Geometry: final body of the model. Coordinates: model frame, mm. A direction names the side the tool comes from. Round coordinates to 2 decimals unless told otherwise and drop trailing zeros. Order: outer loops, then holes, each group sorted by start corner. A loop starts at its lowest first (then second) coordinate and runs counter-clockwise, first axis right, second up. Notation, with made-up numbers: (-3, 28.5) - (24, 28.5) arc R19 ccw to (24, 63.5) - close; hole circle Ø8 at (-33.75, -24). An arc over 180 degrees is marked (long way). Put each result on its own line as item: value. Start each with the question number.
(1) Section B-B (z = 38). Output: boundary loops of the cut face in (x, y), and give its area (3 significant figures).
(2) Section C-C (z = 94). Output: boundary loops of the cut face in (x, y).
(3) Material intervals for L1, parallel to Z at x = 0.85, y = 9.5; L2, parallel to Y at x = 0.55, z = 2.5; L3, parallel to Y at x = 1.45, z = 10, sorted ascending. Write a range as [from, to].
(4) Section D-D (x = 0.8). Count the separate pieces of the cut face and the enclosed holes in it, and give its area (3 significant figures).
(5) Pin query (flat end, axial travel): P1, Ø1.3, axis at x = 1, z = 83, coming from the +Y side; P2, Ø0.8, axis at x = 1, z = 29, coming from the +Y side; P3, Ø0.8, axis at x = 1.5, z = 72, coming from the -Y side. Return the tip coordinate at first contact, or that it passes through.
(6) Access query for faces 1 (the face through (1, 32.105, 83)), 2 (the face through (1, -24, -3.819)), 3 (the face through (1, 33.231, 82)), 4 (the face through (1, -28, 21.581)). Directions: +Z, -Z, +X, -X, +Y, -Y. A direction counts if a zero-diameter tool reaches every point of the face in a straight line with its end or side. Return the directions, or none.
(7) Pull-direction query (Y, two-part tool) for faces 5 (the face through (1.288, 30.863, 106.352)), 6 (the face through (0, -39, 86)), 7 (the face through (1.252, 33.159, -2.864)); classes: released by +Y, released by -Y, zero draft, split by the parting line, or undercut.
(8) Section A-A (y = -12.5). Output: boundary loops of the cut face in (x, z), and give its area (3 significant figures).
Autodesk Inventor part; units mm, degrees
ref_plane "YZ Plane" through (0, 0, 0) normal (1, 0, 0) x (0, 1, 0)
ref_plane "XZ Plane" through (0, 0, 0) normal (0, 1, 0) x (-1, 0, 0)
ref_plane "XY Plane" through (0, 0, 0) normal (0, 0, 1) x (1, 0, 0)
sketch "Sketch1" plane through (0, 0, 0) normal (1, 0, 0) x (0, 1, 0)
  circle A0 centre (30.8347, 52.4486) radius 6.35
  line L0 (34.0644, 46.9813) -> (34.0644, -0.6437)
  line L1 (33.2311, 58.3291) -> (33.2311, 105.9541)
  line L2 (30.0561, 109.1291) -> (27.0711, 109.1291)
  arc A1 (33.2311, 105.9541) -> (30.0561, 109.1291) centre (30.0561, 105.9541) ccw
  line L3 (30.8894, -3.8187) -> (26.3644, -3.8187)
  arc A2 (30.8894, -3.8187) -> (34.0644, -0.6437) centre (30.8894, -0.6437) ccw
  line L4 (27.0711, 109.1291) -> (27.0711, 57.5631)
  line L5 (26.3644, -3.8187) -> (26.3644, 47.9388)
  line L6 (27.0711, 109.1291) -> (27.0711, 83.7291)
  line L7 (27.0711, 109.1291) -> (-79.6089, 109.1291)
  line L8 (-79.6089, 109.1291) -> (-79.6089, 83.7291)
  line L9 (-79.6089, 83.7291) -> (27.0711, 83.7291)
  line L10 (26.3644, -3.8187) -> (-80.3156, -3.8187)
  line L11 (-80.3156, -3.8187) -> (-80.3156, 21.5813)
  line L12 (26.3644, -3.8187) -> (26.3644, 21.5813)
  line L13 (26.3644, 21.5813) -> (-80.3156, 21.5813)
  circle A3 centre (30.8347, 52.4486) radius 4.7025
  point P0 (34.0644, -3.8187)
  point P1 (33.2311, 109.1291)
  dimension "d3" = 50.8
  dimension "d4" = 50.8
  dimension "d5" = 6.16
  dimension "d6" = 3.175
  dimension "d7" = 3.175
  dimension "d8" = 25.4
  dimension "d9" = 106.68
  dimension "d10" = 106.68
  dimension "d11" = 25.4
  dimension "d13" = 25.4
  dimension "d46" = 12.7
extrude "Extrusion1" add sketch "Sketch1" along normal blind 2.54 contours A0 | A0 L4 L2 A1 L1 | L0 A2 L3 L5 A0
sketch "Sketch2" plane through (2.54, 0, 0) normal (1, 0, 0) x (0, 0, -1)
  line L0 (-109.1291, 27.0711) -> (-57.5631, 27.0711)
  line L1 (-109.1291, 27.0711) -> (-109.1291, -79.6089)
  line L2 (-109.1291, -79.6089) -> (-83.7291, -79.6089)
  line L3 (-83.7291, -79.6089) -> (-83.7291, 27.0711)
  line L4 (-109.1291, 27.0711) -> (-83.7291, 27.0711)
  line L5 (3.8187, 26.3644) -> (3.8187, 30.8894)
  line L6 (3.8187, 26.3644) -> (3.8187, -80.3156)
  line L7 (3.8187, -80.3156) -> (-21.5813, -80.3156)
  line L8 (-21.5813, -80.3156) -> (-21.5813, 26.3644)
  line L9 (-47.9388, 26.3644) -> (3.8187, 26.3644)
  point P0 (0, 0)
  dimension "d16" = 106.68
  dimension "d17" = 25.4
  dimension "d18" = 106.68
  dimension "d19" = 25.4
extrude "Extrusion2" add sketch "Sketch2" against normal up to surface (2.54 mm away)
sketch "Sketch3" plane through (2.54, 0, 0) normal (1, 0, 0) x (0, 0, -1)
  line L0 (-83.7291, -79.6089) -> (-83.7291, 27.0711)
  line L1 (-58.3291, 33.2311) -> (-105.9541, 33.2311)
  line L2 (-109.1291, 30.0561) -> (-109.1291, -79.6089)
  line L3 (-109.1291, -79.6089) -> (-83.7291, -79.6089)
  line L4 (-96.4291, 20.7211) -> (-96.4291, 20.7211)
  line L5 (-90.0791, 14.3711) -> (-90.0791, -66.9089)
  line L6 (-96.4291, -73.2589) -> (-96.4291, -73.2589)
  line L7 (-102.7791, -66.9089) -> (-102.7791, 14.3711)
  arc A0 (-96.4291, 20.7211) -> (-102.7791, 14.3711) centre (-96.4291, 14.3711) ccw
  arc A1 (-90.0791, 14.3711) -> (-96.4291, 20.7211) centre (-96.4291, 14.3711) ccw
  arc A2 (-102.7791, -66.9089) -> (-96.4291, -73.2589) centre (-96.4291, -66.9089) ccw
  arc A3 (-96.4291, -73.2589) -> (-90.0791, -66.9089) centre (-96.4291, -66.9089) ccw
  line L8 (-8.8813, 20.0144) -> (-8.8813, 20.0144)
  line L9 (-15.2313, 13.6644) -> (-15.2313, -67.6156)
  line L10 (-8.8813, -73.9656) -> (-8.8813, -73.9656)
  line L11 (-2.5313, -67.6156) -> (-2.5313, 13.6644)
  line L12 (-21.5813, -80.3156) -> (3.8187, -80.3156)
  line L13 (-47.9388, 26.3644) -> (-21.5813, 26.3644)
  line L14 (3.8187, -80.3156) -> (3.8187, 30.8894)
  line L15 (-21.5813, 26.3644) -> (-21.5813, -80.3156)
  arc A4 (-8.8813, 20.0144) -> (-15.2313, 13.6644) centre (-8.8813, 13.6644) ccw
  arc A5 (-2.5313, 13.6644) -> (-8.8813, 20.0144) centre (-8.8813, 13.6644) ccw
  arc A6 (-15.2313, -67.6156) -> (-8.8813, -73.9656) centre (-8.8813, -67.6156) ccw
  arc A7 (-8.8813, -73.9656) -> (-2.5313, -67.6156) centre (-8.8813, -67.6156) ccw
  circle A8 centre (-52.4486, 30.8347) radius 4.7025
  line L16 (-57.1511, 30.8347) -> (-59.6911, 30.8347)
  arc A9 (-59.6911, 29.5647) -> (-59.6911, 32.1047) centre (-59.6911, 30.8347) ccw
  line L17 (-107.6225, 30.8347) -> (-105.0825, 30.8347)
  arc A10 (-105.0825, 32.1047) -> (-105.0825, 29.5647) centre (-105.0825, 30.8347) ccw
  line L18 (-105.0825, 32.1047) -> (-59.6911, 32.1047)
  line L19 (-105.0825, 29.5647) -> (-59.6911, 29.5647)
  line L20 (-47.7461, 30.8347) -> (-45.2061, 30.8347)
  arc A11 (-45.2061, 32.1047) -> (-45.2061, 29.5647) centre (-45.2061, 30.8347) ccw
  arc A12 (0.1852, 29.5647) -> (0.1852, 32.1047) centre (0.1852, 30.8347) ccw
  line L21 (0.1852, 32.1047) -> (-45.2061, 32.1047)
  line L22 (-45.2061, 29.5647) -> (0.1852, 29.5647)
  point P0 (0, 0)
  point P1 (-8.8813, 20.0144)
  point P2 (-8.8813, -73.9656)
  dimension "d26" = 6.35
  dimension "d27" = 6.35
  dimension "d28" = 6.35
  dimension "d29" = 6.35
  dimension "d30" = 6.35
  dimension "d31" = 6.35
  dimension "d32" = 6.35
  dimension "d33" = 6.35
  dimension "d34" = 6.35
  dimension "d35" = 6.35
  dimension "d36" = 2.54
  dimension "d37" = 2.54
  dimension "d38" = 2.54
  dimension "d39" = 2.54
  dimension "d40" = 2.54
  dimension "d41" = 2.54
  dimension "d43" = 2.54
extrude "Extrusion3" cut sketch "Sketch3" against normal through all contours L5 A3 A2 L7 A0 A1 | A4 A5 L11 A7 A6 L9 | L19 A10 L18 A9 | L21 A12 L22 A11
properties part number "Monitor Part ReDes"
Checks:
1. outline: (0, 26.36) - (2.54, 26.36) - (2.54, 29.56) - (0, 29.56) - close; (0, 32.1) - (2.54, 32.1) - (2.54, 34.06) - (0, 34.06) - close
1. area: 13.1 mm²
2. outline: (0, -79.61) - (2.54, -79.61) - (2.54, -72.78) - (0, -72.78) - close; (0, 20.24) - (2.54, 20.24) - (2.54, 29.56) - (0, 29.56) - close; (0, 32.1) - (2.54, 32.1) - (2.54, 33.23) - (0, 33.23) - close
3. L1: z = [-3.82, 2.53], [15.23, 21.58], [83.73, 90.08], [102.78, 109.13]
3. L2: y = [-80.32, 29.56], [32.1, 34.06]
3. L3: y = [-80.32, -73.87], [19.92, 29.56], [32.1, 34.06]
4. separate pieces: 1
4. enclosed holes: 5
4. area: 3,610 mm²
5. P1: stops at y = 33.23
5. P2: stops at y = 34.06
5. P3: stops at y = 27.07
6. face 1: +X, -X
6. face 2: -Z, +X, -X, +Y, -Y
6. face 3: +Z, +X, -X, +Y
6. face 4: +X, -X, -Y
7. face 5: undercut
7. face 6: zero draft
7. face 7: released by +Y
8. outline: (0, -3.82) - (2.54, -3.82) - (2.54, 2.53) - (0, 2.53) - close; (0, 15.23) - (2.54, 15.23) - (2.54, 21.58) - (0, 21.58) - close; (0, 83.73) - (2.54, 83.73) - (2.54, 90.08) - (0, 90.08) - close; (0, 102.78) - (2.54, 102.78) - (2.54, 109.13) - (0, 109.13) - close
8. area: 64.5 mm²
